from build123d import *

# Parameters (mm, degrees)
SKETCH1_W                   = 58.547
SKETCH1_H                   = 44.577
SKETCH1_W_2                 = 47.625
SKETCH1_H_2                 = 26.797
BOSS_EXTRUDE1_DEPTH         = 5.715
BOSS_EXTRUDE2_REACH         = 57.19
SKETCH9_W                   = 1.5875
SKETCH9_H                   = 1.5875
FILLET11_R                  = 3.81
FILLET12_R                  = 3.81
SKETCH21_R                  = 2.54
CUT_EXTRUDE3_DEPTH          = 1.27
F_1_4_CLEARANCE_HOLE1_D     = 6.7564
F_1_4_CLEARANCE_HOLE1_DEPTH = 8.89
F_1_4_CLEARANCE_HOLE1_TIP   = 2.029827343
F_6_32_TAPPED_HOLE1_D       = 2.7051
SKETCH22_W                  = 58.547
SKETCH22_H                  = 7.441182991
CUT_EXTRUDE4_DEPTH          = 41.791028045
FILLET13_R                  = 11.43
FILLET14_R                  = 11.43


with BuildPart() as part:
    # Sketch1 → Boss-Extrude1 (new, symmetric)
    with BuildSketch(Plane(origin=(0, 0, 0), x_dir=(0, 0, -1), z_dir=(1, 0, 0))):
        with Locations((2.921, 0)):
            Rectangle(SKETCH1_W, SKETCH1_H)
        Rectangle(SKETCH1_W_2, SKETCH1_H_2, mode=Mode.SUBTRACT)
    extrude(amount=BOSS_EXTRUDE1_DEPTH, both=True)

    # Sketch9 → Boss-Extrude2 (add, up to next)
    with BuildSketch(Plane.XY.offset(-23.8125), mode=Mode.PRIVATE) as boss_extrude2_sk1:
        with Locations((-4.92125, 12.60475)):
            Rectangle(SKETCH9_W, SKETCH9_H)
    boss_extrude2_tool1 = extrude(boss_extrude2_sk1.sketch, amount=BOSS_EXTRUDE2_REACH, mode=Mode.PRIVATE) - part.part
    # Sketch9 → Boss-Extrude2 (add, up to next)
    with BuildSketch(Plane.XY.offset(-23.8125), mode=Mode.PRIVATE) as boss_extrude2_sk2:
        with Locations((-4.92125, -12.60475)):
            Rectangle(SKETCH9_W, SKETCH9_H)
    boss_extrude2_tool2 = extrude(boss_extrude2_sk2.sketch, amount=BOSS_EXTRUDE2_REACH, mode=Mode.PRIVATE) - part.part
    add(boss_extrude2_tool1.solids().sort_by_distance((-4.92125, 12.60475, -23.8125))[0])
    add(boss_extrude2_tool2.solids().sort_by_distance((-4.92125, -12.60475, -23.8125))[0])

    # Fillet11
    fillet11_edges = [part.edges().sort_by_distance(p)[0] for p in [
        (-4.92125, -11.811, 23.8125),
        (-4.92125, -11.811, -23.8125),
        (-4.92125, 11.811, 23.8125),
        (-4.92125, 11.811, -23.8125),
    ]]
    fillet(fillet11_edges, radius=FILLET11_R)

    # Fillet12
    fillet12_edges = [part.edges().sort_by_distance(p)[0] for p in [
        (0.79375, 13.3985, 23.8125),
        (0.79375, -13.3985, 23.8125),
        (0.79375, -13.3985, -23.8125),
        (0.79375, 13.3985, -23.8125),
    ]]
    fillet(fillet12_edges, radius=FILLET12_R)

    # Sketch21 → Cut-Extrude3 (cut)
    with BuildSketch(Plane(origin=(5.715, 0, 0), x_dir=(0, 0, -1), z_dir=(1, 0, 0))):
        with Locations((33.4645, 9.5885)):
            Circle(SKETCH21_R)
    extrude(amount=-CUT_EXTRUDE3_DEPTH, mode=Mode.SUBTRACT)

    # 1/4 Clearance Hole1
    with Locations(Plane(origin=(-2.530789808, 6.493019647, -32.1945), x_dir=(1, 0, 0), z_dir=(0, 0, -1))):
        with Locations((2.530789808, 13.922519647)):
            Hole(F_1_4_CLEARANCE_HOLE1_D / 2, depth=F_1_4_CLEARANCE_HOLE1_DEPTH)
            with Locations((0, 0, -(F_1_4_CLEARANCE_HOLE1_DEPTH + F_1_4_CLEARANCE_HOLE1_TIP / 2))):  # 118° drill point
                Cone(0, F_1_4_CLEARANCE_HOLE1_D / 2, F_1_4_CLEARANCE_HOLE1_TIP, mode=Mode.SUBTRACT)

    # #6-32 Tapped Hole1 (through all)
    with Locations(Plane(origin=(5.715, 17.955600219, 19.212274833), x_dir=(0, 0, 1), z_dir=(1, 0, 0))):
        with Locations((-27.657774833, 0.175600219), (-16.608774833, 0.175600219), (-5.559774833, 0.175600219), (-38.706774833, 0.175600219), (-38.706774833, 35.735600219), (-27.657774833, 35.735600219), (-16.608774833, 35.735600219), (-5.559774833, 35.735600219)):
            Hole(F_6_32_TAPPED_HOLE1_D / 2)

    # Sketch22 → Cut-Extrude4 (cut, through all)
    with BuildSketch(Plane(origin=(5.715, 0, 0), x_dir=(0, 0, -1), z_dir=(1, 0, 0))):
        with Locations((2.921, -24.485091496)):
            Rectangle(SKETCH22_W, SKETCH22_H)
    extrude(amount=-CUT_EXTRUDE4_DEPTH, mode=Mode.SUBTRACT)

    # Fillet13
    # the kernel refuses this fillet: 11.43 mm, written as the material it takes off along each edge
    with BuildSketch(Plane(origin=(34.29, 22.2885, -32.1945), x_dir=(0, -1, 0), z_dir=(-1, 0, 0)), Plane(origin=(34.29, -20.7645, -32.1945), x_dir=(0, 0, 1), z_dir=(-1, 0, 0))) as fillet13_piece_1:
        with BuildLine():
            CenterArc((FILLET13_R, FILLET13_R), FILLET13_R, 180, 90)
            Line((0, FILLET13_R), (0, 0))
            Line((0, 0), (FILLET13_R, 0))
        make_face()
    extrude(amount=68.58, mode=Mode.SUBTRACT)

    # Fillet14
    fillet14_edges = [part.edges().sort_by_distance(p)[0] for p in [
        (0, -20.7645, 26.3525),
        (0, 22.2885, 26.3525),
    ]]
    fillet(fillet14_edges, radius=FILLET14_R)


solid = part.part
Work out the finished part from the listing and answer in its coordinate system (mm). A direction names the side the tool comes from. Give positions to 0.01 mm unless a question says otherwise; leave off trailing zeros. Loops run counter-clockwise (first coordinate to the right, second up) from the corner with the lowest first, then second, coordinate; pieces in that order, holes last. Notation, with made-up numbers: (-24.75, 46) - (-11.75, 46) arc R16 ccw to (-11.75, 68) - close; hole circle Ø9 at (65, -10). An arc over 180 degrees is marked (long way). Answer in a Markdown table with one row per item.
(1) Flat-ended cylindrical pins translate along their axes: pin 1 Ø4.5 at (y, z) = (10.5, 5) entering from +X; pin 2 Ø3 at (x, z) = (3, -25) entering from +Y. Find the tip coordinate at first contact, or state that the pin passes through.
Results list:
| item | result |
|---|---|
| pin 1 | stops at x = -4.13 |
| pin 2 | stops at y = 21.96 |
(2) Section C-C (x = -5) is taken. State how many separate pieces and enclosed holes the cut face has, and give its area (3 significant figures).
Results list:
| item | result |
|---|---|
| separate pieces | 1 |
| enclosed holes | 9 |
| area | 1,250 mm² |
(3) Section D-D (y = -17.78) is taken. Give the vertices of the cut face in (x, z) (3 decimals).
Results list:
| item | result |
|---|---|
| outline | (-5.715, -28.466) - (5.715, -28.466) - (5.715, -20.847) - (-5.715, -20.847) - close; (-5.715, -18.142) - (5.715, -18.142) - (5.715, -9.798) - (-5.715, -9.798) - close; (-5.715, -7.093) - (5.715, -7.093) - (5.715, 1.251) - (-5.715, 1.251) - close; (-5.715, 3.956) - (5.715, 3.956) - (5.715, 12.3) - (-5.715, 12.3) - close; (-5.715, 15.005) - (5.715, 15.005) - (5.715, 22.624) - (-5.715, 22.624) - close |
(4) Consider L1, parallel to Z at x = -3.5, y = -7; L2, parallel to Y at x = -3.75, z = -15.5; L3, parallel to Y at x = 2.5, z = 15.5. Determine where each line is inside the solid, lowest interval first. Write a range as [from, to].
Results list:
| item | result |
|---|---|
| L1 | z = [-32.19, -23.81], [23.81, 26.35] |
| L2 | y = [-20.76, -13.4], [13.4, 22.29] |
| L3 | y = [-20.75, -13.4], [13.4, 22.27] |
(5) Section A-A (z = 0) is taken. Give the vertices of the cut face in (x, y) (1 decimal).
Results list:
| item | result |
|---|---|
| outline | (-5.7, -20.8) - (5.7, -20.8) - (5.7, -13.4) - (-4.1, -13.4) - (-4.1, -11.8) - (-5.7, -11.8) - close; (-5.7, 11.8) - (-4.1, 11.8) - (-4.1, 13.4) - (5.7, 13.4) - (5.7, 22.3) - (-5.7, 22.3) - close |
(6) Section B-B (y = -1) is taken. Give the vertices of the cut face in (x, z) (1 decimal), and give its area (3 significant figures).
Results list:
| item | result |
|---|---|
| outline | (-5.7, -32.2) - (5.7, -32.2) - (5.7, -23.8) - (-5.7, -23.8) - close; (-5.7, 23.8) - (5.7, 23.8) - (5.7, 26.4) - (-5.7, 26.4) - close |
| area | 125 mm² |
(7) A tool of negligible diameter and unlimited length cuts with its end or side. For faces 4 (the face through (-4.91, 10.72, -22.67)), 5 (the face through (-4.127, 12, 0)), 6 (the face through (0.73, -4.13, -27.84)), 7 (the face through (4.445, 10, -32)), from which of +Z, -Z, +X, -X, +Y, -Y can it reach the whole face along a straight path? Write none if from no direction.
Results list:
| item | result |
|---|---|
| face 4 | +X, -X |
| face 5 | +X |
| face 6 | -Z |
| face 7 | -Z, +X |
(8) For a pull along Y with two mould halves and no side action, classify faces 1 (the face through (0, 1, -32.194)), 2 (the face through (5.089, 9.604, -30.925)), 3 (the face through (0, 22.288, -3)) as pulls with the +Y half, pulls with the -Y half, needs draft (parallel to the pull), parting line crosses it, or undercut.
Results list:
| item | result |
|---|---|
| face 1 | needs draft |
| face 2 | undercut |
| face 3 | pulls with the +Y half |
